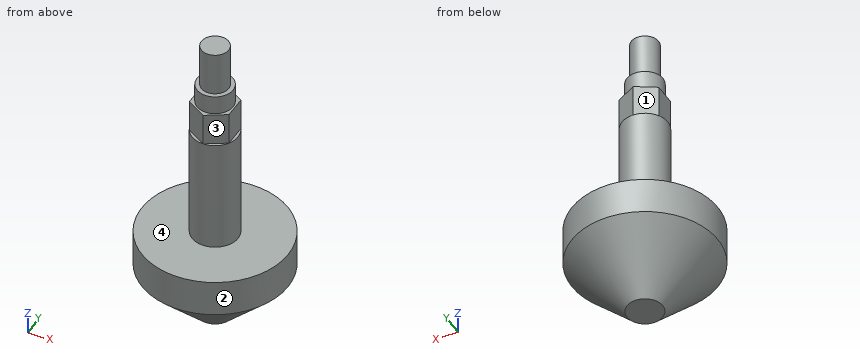
```python
from build123d import *

# Parameters (mm, degrees)
F0_R     = 15.88
F0_R_2   = 10.66
F0_R_3   = 5
F0_R_4   = 3.93
F0_R_5   = 2.975
F1_DEPTH = 20
F2_DEPTH = 45.24
F3_DEPTH = 52.33
F4_DEPTH = 56.5
F5_DEPTH = 66.08
F7_SIZE  = 12


# Not quite as in the source:
# - a feature names something its author has since deleted; it is built from what else it names


with BuildPart() as f1:
    # F0 (on Top) → F1 (new body)
    with BuildSketch(Plane.XY):
        Circle(F0_R)
        Circle(F0_R_2, mode=Mode.SUBTRACT)
        Circle(F0_R_2)
        Circle(F0_R_3, mode=Mode.SUBTRACT)
        Circle(F0_R_3)
        Polygon((0, 4.9883063258), (4.32, 2.4941531629), (4.32, -2.4941531629), (0, -4.9883063258), (-4.32, -2.4941531629), (-4.32, 2.4941531629), align=None, mode=Mode.SUBTRACT)
        Polygon((4.32, -2.4941531629), (4.32, 2.4941531629), (0, 4.9883063258), (-4.32, 2.4941531629), (-4.32, -2.4941531629), (0, -4.9883063258), align=None)
        Circle(F0_R_4, mode=Mode.SUBTRACT)
        Circle(F0_R_4)
        Circle(F0_R_5, mode=Mode.SUBTRACT)
        Circle(F0_R_5)
    extrude(amount=F1_DEPTH)

    # F0 (on Top) → F2 (join)
    with BuildSketch(Plane.XY):
        Circle(F0_R_3)
        Polygon((0, 4.9883063258), (4.32, 2.4941531629), (4.32, -2.4941531629), (0, -4.9883063258), (-4.32, -2.4941531629), (-4.32, 2.4941531629), align=None, mode=Mode.SUBTRACT)
        Polygon((4.32, -2.4941531629), (4.32, 2.4941531629), (0, 4.9883063258), (-4.32, 2.4941531629), (-4.32, -2.4941531629), (0, -4.9883063258), align=None)
        Circle(F0_R_4, mode=Mode.SUBTRACT)
        Circle(F0_R_4)
        Circle(F0_R_5, mode=Mode.SUBTRACT)
        Circle(F0_R_5)
    extrude(amount=F2_DEPTH)

    # F0 (on Top) → F3 (join)
    with BuildSketch(Plane.XY):
        Polygon((4.32, -2.4941531629), (4.32, 2.4941531629), (0, 4.9883063258), (-4.32, 2.4941531629), (-4.32, -2.4941531629), (0, -4.9883063258), align=None)
        Circle(F0_R_4, mode=Mode.SUBTRACT)
        Circle(F0_R_4)
        Circle(F0_R_5, mode=Mode.SUBTRACT)
        Circle(F0_R_5)
    extrude(amount=F3_DEPTH)

    # F0 (on Top) → F4 (join)
    with BuildSketch(Plane.XY):
        Circle(F0_R_4)
        Circle(F0_R_5, mode=Mode.SUBTRACT)
        Circle(F0_R_5)
    extrude(amount=F4_DEPTH)

    # F0 (on Top) → F5 (join)
    with BuildSketch(Plane.XY):
        Circle(F0_R_5)
    extrude(amount=F5_DEPTH)

    # F7
    f7_edges = [f1.edges().sort_by_distance(p)[0] for p in [
        (-15.88, 0, 0),
    ]]
    chamfer(f7_edges, length=F7_SIZE)


solid = f1.part
```
Geometry: final body of the model. Coordinates: model frame, mm. Face numbers are marked on the shaded views. A direction names the side the tool comes from. Coordinates: 2 decimals unless noted, no trailing zeros. Order: outer loops, then holes, each group sorted by start corner. A loop starts at its lowest first (then second) coordinate and runs counter-clockwise, first axis right, second up. Notation, with made-up numbers: (21.25, 67.25) - (25.25, 67.25) arc R15 cw to (25.25, 96.25) - close; hole circle Ø6 at (-20, -38). An arc over 180 degrees is marked (long way). Write each question's results on one line, items separated by ' | '.
1) Line query: line 1 (X direction, y = -1, z = 51.5); line 2 (Y direction, x = -4, z = 6); line 3 (X direction, y = 3.5, z = 8.5). Output: solid intervals per line, ascending. Write a range as from..to.
Results list:
line 1: -4.32..4.32 | line 2: -9.03..9.03 | line 3: -11.87..11.87
2) Pin query (flat end, axial travel): pin 1 (5 mm diameter, centred on x = -7.5, z = 46, fed in from +Y); pin 2 (6 mm diameter, centred on y = -1.5, z = 37.5, fed in from +X); pin 3 (1 mm diameter, centred on y = 8, z = 17, fed in from +X); pin 4 (1.5 mm diameter, centred on x = -6.5, y = -9, fed in from +Z). Return the tip coordinate at first contact, or that it passes through.
Results list:
pin 1: through | pin 2: x = 5 | pin 3: x = 14 | pin 4: z = 20
3) Section A-A, the plane y = 0. Return loops of the section in (x, z) (3 decimals), plus the area to 3 significant figures.
Results list:
outline: (-15.88, 12) - (-3.88, 0) - (3.88, 0) - (15.88, 12) - (15.88, 20) - (5, 20) - (5, 45.24) - (4.32, 45.24) - (4.32, 52.33) - (3.93, 52.33) - (3.93, 56.5) - (2.975, 56.5) - (2.975, 66.08) - (-2.975, 66.08) - (-2.975, 56.5) - (-3.93, 56.5) - (-3.93, 52.33) - (-4.32, 52.33) - (-4.32, 45.24) - (-5, 45.24) - (-5, 20) - (-15.88, 20) - close | area: 895 mm^2
4) Section C-C, the plane z = 7.5. Return loops of the section in (x, y).
Results list:
outline: circle Ø22.76 at (0, 0)
5) Set-up query: the marked faces 1, 2, 3 and 4. Return all of +Z, -Z, +X, -X, +Y, -Y with unobstructed straight access to the full face (end or side cutting, diameter ignored); none if empty.
Results list:
face 1: +Z, -X, +Y | face 2: +Z, -Z | face 3: +Z, +X, -Y | face 4: +Z
6) Section B-B, the plane z = 38.5. Return loops of the section in (x, y), plus the area to 3 significant figures.
Results list:
outline: circle Ø10 at (0, 0) | area: 78.5 mm^2
